```python
from build123d import *

# Parameters (mm, degrees)
SKETCH1_W                    = 104.78
SKETCH1_H                    = 53.63
BOSS_EXTRUDE1_DEPTH          = 6.35
F_30_0_1285_DIAMETER_HOLE1_D = 3.2639
F_0_257_DIAMETER_HOLE1_D     = 6.5278
FILLET1_R                    = 5


with BuildPart() as part:
    # Sketch1 → Boss-Extrude1 (new body)
    with BuildSketch(Plane(origin=(0, 0, 0), x_dir=(1, 0, 0), z_dir=(0, 1, 0))):
        with Locations((52.39, 26.815)):
            Rectangle(SKETCH1_W, SKETCH1_H)
    extrude(amount=BOSS_EXTRUDE1_DEPTH)

    # #30 (0.1285) Diameter Hole1 (through all)
    with Locations(Plane(origin=(0, 0, 0), x_dir=(-1, 0, 0), z_dir=(0, -1, 0))):
        with Locations((-98.43, 7.765), (-98.43, 45.865), (-74.6175, 7.765), (-74.6175, 45.865), (-30.1675, 7.765), (-30.1675, 45.865), (-6.355, 7.765), (-6.355, 45.865)):
            Hole(F_30_0_1285_DIAMETER_HOLE1_D / 2)

    # F (0.257) Diameter Hole1 (through all)
    with Locations(Plane(origin=(0, 0, 0), x_dir=(-1, 0, 0), z_dir=(0, -1, 0))):
        with Locations((-52.39, 26.815)):
            Hole(F_0_257_DIAMETER_HOLE1_D / 2)

    # Fillet1
    fillet1_edges = [part.edges().sort_by_distance(p)[0] for p in [
        (0, 3.175, -53.63),
        (104.78, 3.175, -53.63),
        (104.78, 3.175, 0),
        (0, 3.175, 0),
    ]]
    fillet(fillet1_edges, radius=FILLET1_R)


solid = part.part
```
Work out the finished part from the listing and answer in its coordinate system (mm). Coordinates: 2 decimals unless noted, no trailing zeros. Write each loop counter-clockwise with the first axis right and the second up, starting at its lowest first coordinate (ties: lowest second). Pieces come first, ordered by that corner, then holes.
Q1. A cutting plane is placed at A-A, the plane x = 52.39. Give the vertices of the cut face in (y, z), then the cut area to 3 significant figures.
Q2. Find the intervals of material crossed by line 1 (X direction, y = 1, z = -8); line 2 (X direction, y = 6, z = -46.5); line 3 (Z direction, x = 52.39, y = 5.25), in increasing order.
Q3. Determine the mould class of faces 1 (the face through (30.921, 3.219, -44.417)), 2 (the face through (0, 3, -27)), 3 (the face through (103.28, 3.22, -52.2)), 4 (the face through (31.724, 3.219, -8.255)) for opening direction Z: released by +Z, released by -Z, zero draft, split by the parting line, or undercut.
Q4. A cutting plane is placed at B-B, the plane x = 98.43. Give the vertices of the cut face in (y, z), then the cut area to 3 significant figures.
Q5. A cutting plane is placed at C-C, the plane y = 3.5. State how many separate pieces and enclosed holes the cut face has, then the cut area to 3 significant figures.
Findings below:
1. outline: (0, -53.63) - (6.35, -53.63) - (6.35, -30.08) - (0, -30.08) - close; (0, -23.55) - (6.35, -23.55) - (6.35, 0) - (0, 0) - close
1. area: 299 mm2
2. line 1: x = 0 to 4.74, 7.97 to 28.55, 31.78 to 73, 76.23 to 96.82, 100.04 to 104.78
2. line 2: x = 0 to 4.85, 7.86 to 28.66, 31.67 to 73.11, 76.12 to 96.93, 99.93 to 104.78
2. line 3: z = -53.63 to -30.08, -23.55 to 0
3. face 1: undercut
3. face 2: zero draft
3. face 3: released by -Z
3. face 4: undercut
4. outline: (0, -53.63) - (6.35, -53.63) - (6.35, -47.5) - (0, -47.5) - close; (0, -44.23) - (6.35, -44.23) - (6.35, -9.4) - (0, -9.4) - close; (0, -6.13) - (6.35, -6.13) - (6.35, 0) - (0, 0) - close
4. area: 299 mm2
5. separate pieces: 1
5. enclosed holes: 9
5. area: 5,500 mm2
